from build123d import *

# Parameters (mm, degrees)
SKETCH1_W           = 20
SKETCH1_H           = 33
SKETCH1_R           = 2.15
BOSS_EXTRUDE1_DEPTH = 5
SKETCH2_W           = 20
SKETCH2_H           = 4
BOSS_EXTRUDE2_DEPTH = 38
SKETCH4_W           = 20
SKETCH4_H           = 7.411842069
BOSS_EXTRUDE3_DEPTH = 25
FILLET1_R           = 3
FILLET2_R           = 2
FILLET4_R           = 3
CHAMFER2_SIZE       = 2
SKETCH8_W           = 20
SKETCH8_H           = 5
BOSS_EXTRUDE5_DEPTH = 25.588157931
FILLET7_R           = 3
SKETCH12_W          = 20
SKETCH12_H          = 10
BOSS_EXTRUDE6_DEPTH = 14
SKETCH3_R           = 3.7
CUT_EXTRUDE2_DEPTH  = 15
FILLET8_R           = 3


with BuildPart() as part:
    # Sketch1 → Boss-Extrude1 (new body)
    with BuildSketch(Plane.XY):
        with Locations((10, -16.5)):
            Rectangle(SKETCH1_W, SKETCH1_H)
        with Locations((10, -6.5)):
            Circle(SKETCH1_R, mode=Mode.SUBTRACT)
        with Locations(Location((10, -26.5, 0), (0, 0, 180))):
            Circle(SKETCH1_R, mode=Mode.SUBTRACT)
    extrude(amount=BOSS_EXTRUDE1_DEPTH)

    # Sketch2 → Boss-Extrude2 (add)
    with BuildSketch(Plane(origin=(0, 0, 0), x_dir=(-1, 0, 0), z_dir=(0, 0, -1))):
        with Locations((-10, 2)):
            Rectangle(SKETCH2_W, SKETCH2_H)
    extrude(amount=-BOSS_EXTRUDE2_DEPTH)

    # Sketch4 → Boss-Extrude3 (add)
    with BuildSketch(Plane.XZ):
        with Locations((10, 34.294078965)):
            Rectangle(SKETCH4_W, SKETCH4_H)
    extrude(amount=BOSS_EXTRUDE3_DEPTH)

    # Fillet1
    fillet1_edges = [part.edges().sort_by_distance(p)[0] for p in [
        (20, -10.5, 38),
        (0, -10.5, 38),
    ]]
    fillet(fillet1_edges, radius=FILLET1_R)

    # Fillet2
    fillet2_edges = [part.edges().sort_by_distance(p)[0] for p in [
        (10, -33, 5),
    ]]
    fillet(fillet2_edges, radius=FILLET2_R)

    # Fillet4
    fillet4_edges = [part.edges().sort_by_distance(p)[0] for p in [
        (10, -25, 30.588157931),
    ]]
    fillet(fillet4_edges, radius=FILLET4_R)

    # Chamfer2
    chamfer2_edges = [part.edges().sort_by_distance(p)[0] for p in [
        (10, 0, 5),
    ]]
    chamfer(chamfer2_edges, length=CHAMFER2_SIZE)

    # Sketch8 → Boss-Extrude5 (add)
    with BuildSketch(Plane.XY.offset(5)):
        with Locations((10, -16.5)):
            Rectangle(SKETCH8_W, SKETCH8_H)
    extrude(amount=BOSS_EXTRUDE5_DEPTH)

    # Fillet7
    fillet7_edges = [part.edges().sort_by_distance(p)[0] for p in [
        (10, -19, 5),
        (10, -19, 30.588157931),
        (10, -14, 5),
    ]]
    fillet(fillet7_edges, radius=FILLET7_R - 0.0001)  # a hair under: the kernel refuses the full size

    # Sketch12 → Boss-Extrude6 (add)
    with BuildSketch(Plane(origin=(0, -14, 0), x_dir=(1, 0, 0), z_dir=(0, 1, 0))):
        with Locations((10, -25.588157931)):
            Rectangle(SKETCH12_W, SKETCH12_H)
    extrude(amount=BOSS_EXTRUDE6_DEPTH)

    # Sketch3 → Cut-Extrude2 (cut)
    with BuildSketch(Plane(origin=(0, 4, 0), x_dir=(1, 0, 0), z_dir=(0, 1, 0))):
        with Locations(Location((10, -27, 0), (0, 0, 270))):
            Circle(SKETCH3_R)
    extrude(amount=-CUT_EXTRUDE2_DEPTH, mode=Mode.SUBTRACT)

    # Fillet8
    fillet8_edges = [part.edges().sort_by_distance(p)[0] for p in [
        (10, 0, 20.588157931),
        (10, -14, 20.588157931),
    ]]
    fillet(fillet8_edges, radius=FILLET8_R)


solid = part.part
For this review, take the finished solid that the model builds, in its own axes (mm). A direction names the side the tool comes from. Give positions to 0.01 mm unless a question says otherwise; leave off trailing zeros. Order: outer loops, then holes, each group sorted by start corner. A loop starts at its lowest first (then second) coordinate and runs counter-clockwise, first axis right, second up. Notation, with made-up numbers: M 52.5,-11 L 100.5,-11 A16 cw 100.5,2 Z; hole C -28.5,-27 d5. An arc over 180 degrees is marked long. Answer in a Markdown table with one row per item. Add a question column.
(1) Consider section D-D on z = 27. State the section outline as (x, y) points.
(2) Mouldability with a two-part tool opening along Y and no side actions: class faces 5 (the face through (10, -33, 1)), 6 (the face through (10, -10, 38)), 7 (the face through (10.14, -13.1, 5.86)) as +Y half, -Y half, draft (parallel to the pull), parting line (faces both ways), or undercut.
(3) Consider section A-A on y = -6.5. State the section outline as (x, z) points.
(4) Wall thickness on probe 1 along Y at (x, z) = (10, 2.35); probe 2 along X at (y, z) = (-26.5, 1.3); probe 3 along X at (y, z) = (-4, 27): over which ranges is each line inside the solid? List them lowest first. Write a range as [from, to].
(5) For faces 1 (the face through (7.85, -6.41, 2.46)), 2 (the face through (10.14, -19.9, 29.73)), 3 (the face through (10, -25, 36)), 4 (the face through (10.14, -13.1, 19.73)), list the 3-axis set-ups (+Z, -Z, +X, -X, +Y, -Y) from which the entire face can be reached by the end or side of a thin tool; tool diameter is ignored.
(6) For pin 1 (3.5 mm diameter, centred on x = 9.5, z = 28.5, fed in from +Y); pin 2 (4 mm diameter, centred on x = 5, z = 30.5, fed in from -Y); pin 3 (4 mm diameter, centred on x = 10, y = -6.5, fed in from -Z); pin 4 (1 mm diameter, centred on y = -3, z = 20, fed in from -X), all flat-tipped, find the tip position at first contact; note any pin that passes through.
(7) Consider section C-C on y = -26.5. State the section outline as (x, z) points, and give its area (3 significant figures).
Evaluation:
| question | item | result |
|---|---|---|
| 1 | outline | M 0,-19 L 20,-19 L 20,4 L 13.7,4 L 13.7,-11 L 6.3,-11 L 6.3,4 L 0,4 Z |
| 2 | face 5 | -Y half |
| 2 | face 6 | draft |
| 2 | face 7 | undercut |
| 3 | outline | M 0,0 L 7.85,0 L 7.85,5 L 0,5 Z; M 0,20.59 L 20,20.59 L 20,35 A3 ccw 17,38 L 3,38 A3 ccw 0,35 Z; M 12.15,0 L 20,0 L 20,5 L 12.15,5 Z; hole C 10,27 d7.4 |
| 4 | probe 1 | y = [-33, -28.65], [-24.35, -8.65], [-4.35, 4] |
| 4 | probe 2 | x = [0, 7.85], [12.15, 20] |
| 4 | probe 3 | x = [0, 6.3], [13.7, 20] |
| 5 | face 1 | -Z |
| 5 | face 2 | +X, -X, -Y |
| 5 | face 3 | +Z, +X, -X, -Y |
| 5 | face 4 | +X, -X |
| 6 | pin 1 | stops at y = -11 |
| 6 | pin 2 | stops at y = -24.8 |
| 6 | pin 3 | stops at z = 20.59 |
| 6 | pin 4 | passes through |
| 7 | outline | M 0,0 L 7.85,0 L 7.85,5 L 0,5 Z; M 12.15,0 L 20,0 L 20,5 L 12.15,5 Z |
| 7 | area | 78.5 mm^2 |
